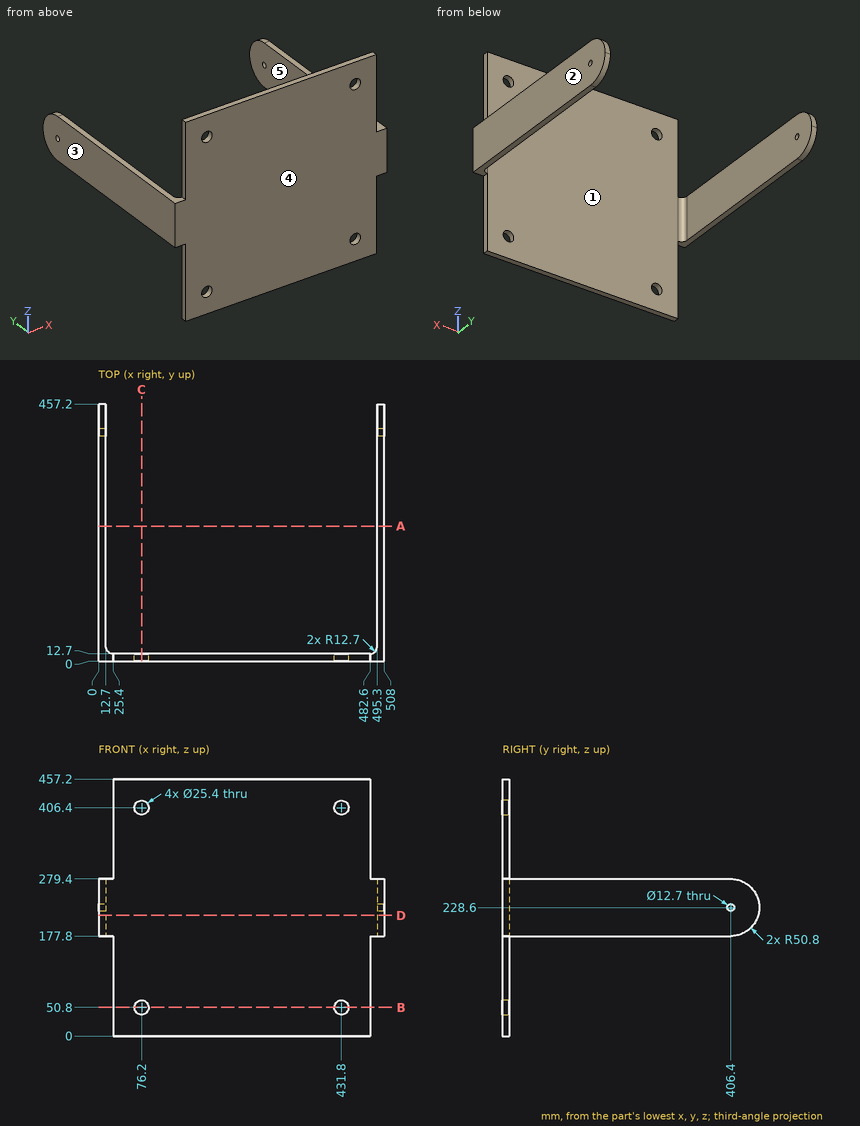
Could you check a few things on this drawing? It's one solid part, dimensions in mm from its lowest x, y, z. A direction names the side the tool comes from. Coordinates: 2 decimals unless noted, no trailing zeros. Loops run counter-clockwise (first coordinate to the right, second up) from the corner with the lowest first, then second, coordinate; pieces in that order, holes last. Notation, with made-up numbers: (50, -26) - (54, -26) arc R31 cw to (54, 5) - close; hole circle Ø5 at (-0.5, 78.25). An arc over 180 degrees is marked (long way). Answer as a JSON object with one key per item and string values. Group by question number.
Item 1: If we mould it in two halves opening along X, with no side actions, what happens to the marked faces 3, 4 and 5? For each: released by +X, released by -X, zero draft, split by the parting line, or undercut.
Item 2: If we section it at A-A (y = 240): List the corners of the cut face in (x, z) for me, plus the area to 3 significant figures.
Item 3: If we section it at C-C (x = 76.2): List the corners of the cut face in (y, z) for me, plus the area to 3 significant figures.
Item 4: On a 3-axis mill with a long thin cutter (end or side, diameter ignored), from which of +Z, -Z, +X, -X, +Y, -Y can I reach the whole of each face in a straight line? I mean the marked faces 1 and 2. Say none if no direction works.
Item 5: If we section it at B-B (z = 50.8): List the corners of the cut face in (x, y) for me.
Item 6: For pin 1 (7.5 mm diameter, centred on x = 493.5, y = 167.5, fed in from -Z); pin 2 (14 mm diameter, centred on y = 4, z = 116, fed in from +X); pin 3 (10 mm diameter, centred on y = 9.5, z = 123, fed in from -X), each with a flat end and sliding along its axis, tell me the tip position at first contact or that it passes through.
Item 7: If we section it at D-D (z = 214.5): List the corners of the cut face in (x, y) for me, plus the area to 3 significant figures.
Item 8: If I drill on L1, parallel to Z at x = 431, y = 4 (3 decimals); L2, parallel to X at y = 6, z = 406; L3, parallel to X at y = 105, z = 248, over which ranges is the centre line in solid material (lowest first)? Write a range as from..to.
Returned:
{
 "1": {"face 3": "released by -X", "face 4": "zero draft", "face 5": "undercut"},
 "2": {"outline": "(0, 177.8) - (12.7, 177.8) - (12.7, 279.4) - (0, 279.4) - close; (495.3, 177.8) - (508, 177.8) - (508, 279.4) - (495.3, 279.4) - close", "area": "2,580 mm²"},
 "3": {"outline": "(0, 0) - (12.7, 0) - (12.7, 38.1) - (0, 38.1) - close; (0, 63.5) - (12.7, 63.5) - (12.7, 393.7) - (0, 393.7) - close; (0, 419.1) - (12.7, 419.1) - (12.7, 457.2) - (0, 457.2) - close", "area": "5,160 mm²"},
 "4": {"face 1": "+Z, -Z, +Y", "face 2": "+Z, -Z, +X, +Y, -Y"},
 "5": {"outline": "(25.4, 0) - (63.5, 0) - (63.5, 12.7) - (25.4, 12.7) - close; (88.9, 0) - (419.1, 0) - (419.1, 12.7) - (88.9, 12.7) - close; (444.5, 0) - (482.6, 0) - (482.6, 12.7) - (444.5, 12.7) - close"},
 "6": {"pin 1": "stops at z = 177.8", "pin 2": "stops at x = 482.6", "pin 3": "stops at x = 25.4"},
 "7": {"outline": "(0, 0) - (508, 0) - (508, 455.2) - (495.3, 455.2) - (495.3, 25.4) arc R12.7 cw to (482.6, 12.7) - (25.4, 12.7) arc R12.7 cw to (12.7, 25.4) - (12.7, 455.2) - (0, 455.2) - close", "area": "17,800 mm²"},
 "8": {"L1": "z = 0..38.125, 63.475..393.725, 419.075..457.2", "L2": "x = 25.4..63.51, 88.89..419.11, 444.49..482.6", "L3": "x = 0..12.7, 495.3..508"}
}
